from build123d import *

# Parameters (mm, degrees)
FILLET1_R    = 1.5
SKETCH3_W    = 1.42
SKETCH3_H    = 7.1
SKETCH4_W    = 1.42
SKETCH4_H    = 3.26092226
RECPAT_COUNT = 2
RECPAT_ANGLE = 90


with BuildPart() as part:
    # BodySke → Base-Revolve (revolve)
    with BuildSketch(Plane.XY):
        with BuildLine():
            Line((0, 0), (61.4, 0))
            Line((61.4, 0), (61.4, 3))
            Line((61.4, 3), (4.7, 3))
            Line((4.7, 3), (2.05, 5.65))
            Line((2.05, 5.65), (1.4, 5.65))
            ThreePointArc((1.4, 5.65), (0.355213526, 2.910433816), (0, 0))
        make_face()
    revolve(axis=Axis((-15.875, 0, 0), (1, 0, 0)))

    # Fillet1
    fillet1_edges = [part.edges().sort_by_distance(p)[0] for p in [
        (4.7, -3, 0),
    ]]
    fillet(fillet1_edges, radius=FILLET1_R)

    # Sketch3 → Recess section 0
    with BuildSketch(Plane(origin=(0, 0, 0), x_dir=(0, 0, -1), z_dir=(1, 0, 0))):
        Rectangle(SKETCH3_W, SKETCH3_H)
    # Sketch4 → Recess section 1
    with BuildSketch(Plane(origin=(3.85, 0, 0), x_dir=(0, 0, -1), z_dir=(1, 0, 0))):
        Rectangle(SKETCH4_W, SKETCH4_H)
    recess = loft(mode=Mode.SUBTRACT)

    # RecPat: Recess ×2 about axis
    recpat_axis = Axis((0, 0, 0), (1, 0, 0))
    for i in range(1, RECPAT_COUNT):
        add(recess.rotate(recpat_axis, i * RECPAT_ANGLE / (RECPAT_COUNT - 1)), mode=Mode.SUBTRACT)

    # RecCorSke → RecessCore (revolve, cut)
    with BuildSketch(Plane.XY):
        Polygon((0, 0), (0, 1.549718226), (3.85, 1.2805), (4.266059671, 0), align=None)
    revolve(axis=Axis((-3.175, 0, 0), (1, 0, 0)), mode=Mode.SUBTRACT)


solid = part.part
CAD build for the part. Positions are in the model's coordinates, mm. A direction names the side the tool comes from. Give positions to 0.01 mm unless a question says otherwise; leave off trailing zeros. Write each loop counter-clockwise with the first axis right and the second up, starting at its lowest first coordinate (ties: lowest second). Pieces come first, ordered by that corner, then holes. Notation, with made-up numbers: M 67.5,-21 L 119.5,-21 A29 cw 119.5,11 Z; hole C -32,81 d9. An arc over 180 degrees is marked long. Put each result on its own line as item: value. Start each with the question number.
(1) Which spindle directions (+Z, -Z, +X, -X, +Y, -Y) get a long thin tool onto all of the face, cutting with end or side? Do faces 1 (the face through (2.181, 2.463, -0.01)), 2 (the face through (32.97, 2.86, 0.9)), 3 (the face through (1.72, 5.39, 1.7)). Say none if no direction does.
(2) Probe L1, parallel to Y at x = 16, z = 0.25; L2, parallel to X at y = 1.5, z = -0.5. List the from-to ranges inside material, lowest first.
(3) Mould opens along Y. For faces 4 (the face through (4.122, 3.305, -1.37)), 5 (the face through (2.181, 0.01, 2.463)), 6 (the face through (61.4, 0, 0)), 7 (the face through (4.246, -0.013, -0.061)) say: +Y half, -Y half, draft (parallel to the pull), parting line (faces both ways), or undercut.
(4) Flat gauge pins, fed straight in: pin 1 Ø5 at (x, z) = (21.5, 0.5) entering from +Y; pin 2 Ø1.5 at (x, y) = (39, 2.5) entering from +Z; pin 3 Ø1.5 at (x, z) = (50.5, 1.5) entering from +Y; pin 4 Ø4 at (y, z) = (-2, -4) entering from +X. Where does each tip first touch, or does it go through?
(5) Band-saw the part on A-A, the plane x = 7. Write the cut outline in (y, z).
Response values:
1. face 1: -X
1. face 2: +X
1. face 3: +X, -X
2. L1: y = -2.99 to 2.99
2. L2: x = 3.85 to 61.4
3. face 4: parting line
3. face 5: undercut
3. face 6: draft
3. face 7: undercut
4. pin 1: stops at y = 3
4. pin 2: stops at z = 2.44
4. pin 3: stops at y = 2.9
4. pin 4: stops at x = 61.4
5. outline: C 0,0 d6
